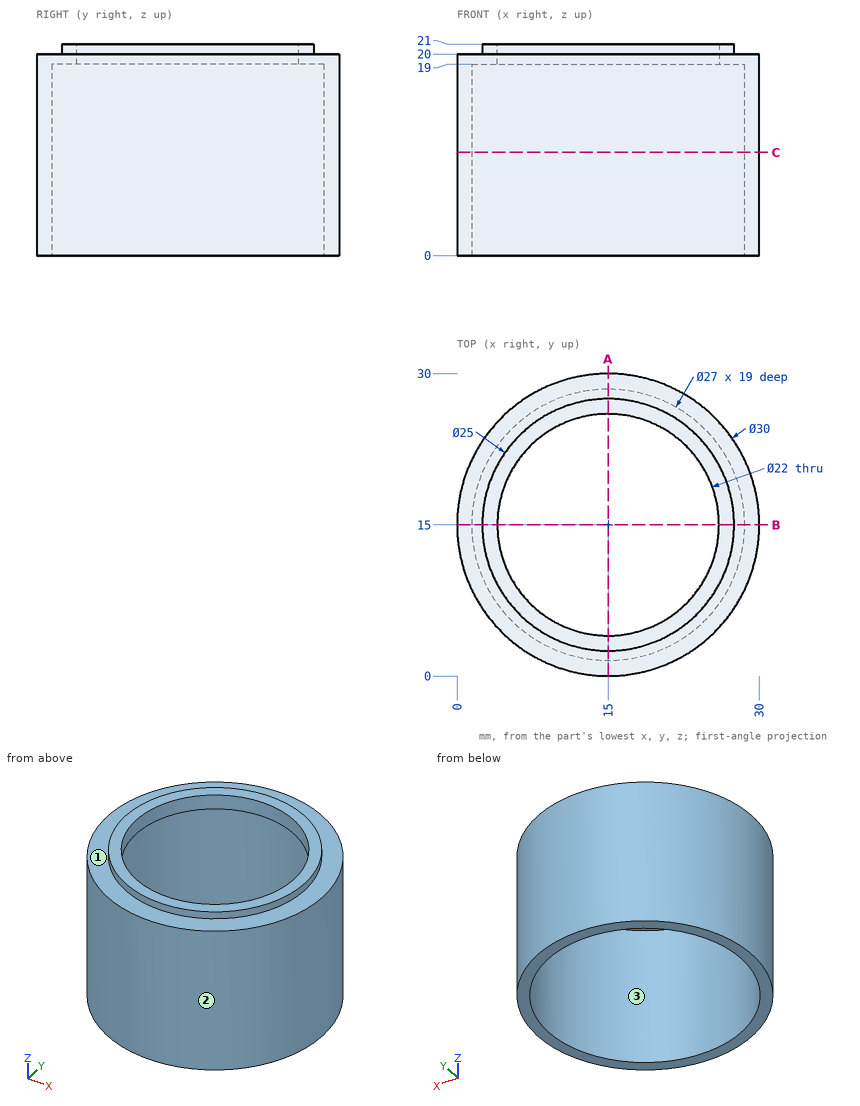
Source: three-view drawing plus pictorial views. Frame: mm from the lowest corner of the part. Coordinates: 2 decimals unless noted, no trailing zeros. Loops run counter-clockwise (first coordinate to the right, second up) from the corner with the lowest first, then second, coordinate; pieces in that order, holes last. Notation, with made-up numbers: (8.25, -26) - (37.25, -26) arc R10 ccw to (37.25, -17) - close; hole circle Ø7 at (-21, -10.75). An arc over 180 degrees is marked (long way). Answer in a Markdown table with one row per item. Add a question column.
Item 1: Section query C-C on z = 10.25. Return the cut outline in (x, y), then the cut area to 3 significant figures.
Item 2: Contact query for flat-ended pins moving along their axis: P1, Ø1, axis at x = 22.5, z = 11.5, coming from the +Y side; P2, Ø4, axis at y = 24, z = 7.5, coming from the +X side; P3, Ø2, axis at x = 13.5, z = 14.5, coming from the -Y side. Output: stop coordinate, or through.
Item 3: Section query A-A on x = 15. Return the cut outline in (y, z).
Item 4: Mould query, pull axis X, two halves, no side actions, for the marked faces 1, 2 and 3. Classes: released by +X, released by -X, zero draft, split by the parting line, or undercut.
Item 5: Line query: line 1 along Y through (x, z) = (15, 19.65); line 2 along Y through (x, z) = (15, 14.5); line 3 along Z through (x, y) = (4, 24.75). Output: solid intervals per line, ascending. Write a range as [from, to].
Recorded:
| question | item | result |
|---|---|---|
| 1 | outline | circle Ø30 at (15, 15); hole circle Ø27 at (15, 15) |
| 1 | area | 134 mm^2 |
| 2 | P1 | y = 28.27 |
| 2 | P2 | x = 28.27 |
| 2 | P3 | y = 0.01 |
| 3 | outline | (0, 0) - (1.5, 0) - (1.5, 19) - (4, 19) - (4, 21) - (2.5, 21) - (2.5, 20) - (0, 20) - close; (26, 19) - (28.5, 19) - (28.5, 0) - (30, 0) - (30, 20) - (27.5, 20) - (27.5, 21) - (26, 21) - close |
| 4 | face 1 | zero draft |
| 4 | face 2 | split by the parting line |
| 4 | face 3 | undercut |
| 5 | line 1 | [0, 4], [26, 30] |
| 5 | line 2 | [0, 1.5], [28.5, 30] |
| 5 | line 3 | [0, 20] |
